```python
from build123d import *

# Parameters (mm, degrees)
BOSS_EXTRUDE1_DEPTH = 3
SKETCH2_W           = 56
SKETCH2_H           = 25
CUT_EXTRUDE1_DEPTH  = 76.013332148


with BuildPart() as part:
    # Sketch1 → Boss-Extrude1 (new body)
    with BuildSketch(Plane(origin=(0, 0, 0), x_dir=(1, 0, 0), z_dir=(0, 1, 0))):
        Polygon((0, -3), (0, 0), (3, 0), (3, 6), (0, 6), (0, 12), (3, 12), (3, 22), (0, 22), (0, 28), (3, 28), (3, 38), (0, 38), (0, 44), (3, 44), (3, 50), (0, 50), (0, 53), (-6, 53), (-6, 50), (-12, 50), (-12, 53), (-22, 53), (-22, 50), (-28, 50), (-28, 53), (-38, 53), (-38, 50), (-44, 50), (-44, 53), (-50, 53), (-50, 44), (-53, 44), (-53, 38), (-50, 38), (-50, 28), (-53, 28), (-53, 22), (-50, 22), (-50, 12), (-53, 12), (-53, 6), (-50, 6), (-50, -3), (-44, -3), (-44, 0), (-38, 0), (-38, -3), (-28, -3), (-28, 0), (-22, 0), (-22, -3), (-12, -3), (-12, 0), (-6, 0), (-6, -3), align=None)
    extrude(amount=BOSS_EXTRUDE1_DEPTH)

    # Sketch2 → Cut-Extrude1 (cut, through all)
    with BuildSketch(Plane(origin=(0, 3, 0), x_dir=(1, 0, 0), z_dir=(0, 1, 0))):
        with Locations((-25, 40.5)):
            Rectangle(SKETCH2_W, SKETCH2_H)
    extrude(amount=-CUT_EXTRUDE1_DEPTH, mode=Mode.SUBTRACT)


solid = part.part
```
Here's how the part is built. I have some questions about the finished solid (model axes, mm). A direction names the side the tool comes from. Coordinates: 2 decimals unless noted, no trailing zeros. Order: outer loops, then holes, each group sorted by start corner. A loop starts at its lowest first (then second) coordinate and runs counter-clockwise, first axis right, second up. Notation, with made-up numbers: (-9.75, -30) -> (48.25, -30) arc R13 cw to (48.25, -11) -> close; hole circle Ø1 at (60, 6). An arc over 180 degrees is marked (long way). Return JSON: item names as keys, results as strings.
1) If I drill on probe 1 along X at (y, z) = (2.7, 2.5); probe 2 along X at (y, z) = (0.6, -13); probe 3 along X at (y, z) = (2.35, -27), over which ranges is the centre line in solid material (lowest first)?
Conclusion:
{"probe 1": "x = -50 to -44, -38 to -28, -22 to -12, -6 to 0", "probe 2": "x = -50 to 3", "probe 3": "x = -53 to 0"}
2) I'm going to push flat-ended pins straight in: P1, Ø1.5, axis at y = 1.5, z = 1, coming from the -X side; P2, Ø0.9, axis at x = 1.5, y = 2, coming from the +Z side; P3, Ø1.5, axis at y = 2, z = 1, coming from the +X side; P4, Ø2, axis at x = -33.5, z = -11, coming from the -Y side. Where does each tip first touch, or does it pass through?
Conclusion:
{"P1": "stops at x = -50", "P2": "stops at z = 0", "P3": "stops at x = 0", "P4": "stops at y = 0"}
3) Thinking about a two-plate mould opening in Z: for faces 1 (the flat face through (-51, 1, -12)), 2 (the flat face through (-44, 1, 2)), 3 (the flat face through (-3, 1, 3)), which applies, +Z half, -Z half, draft (parallel to the pull), parting line (faces both ways), or undercut?
Conclusion:
{"face 1": "undercut", "face 2": "draft", "face 3": "+Z half"}
4) If we section it at B-B on x = -10.5: List the corners of the cut face in (y, z) for me.
Conclusion:
{"outline": "(0, -28) -> (3, -28) -> (3, 0) -> (0, 0) -> close"}
5) If we section it at C-C on z = -2: List the corners of the cut face in (x, y) for me, plus the area to 3 significant figures.
Conclusion:
{"outline": "(-50, 0) -> (3, 0) -> (3, 3) -> (-50, 3) -> close", "area": "159 mm²"}
6) On a 3-axis mill with a long thin cutter (end or side, diameter ignored), from which of +Z, -Z, +X, -X, +Y, -Y can I reach the whole of each face in a straight line? I mean faces 4 (the flat face through (-22, 1, 1)), 5 (the flat face through (0, 1, -25)), 6 (the flat face through (2, 1, -6)). Say none if no direction works.
Conclusion:
{"face 4": "+Z, +Y, -Y", "face 5": "-Z, +X, +Y, -Y", "face 6": "+X, +Y, -Y"}
